CAD build for the part. Positions are in the model's coordinates, mm. Face numbers are marked on the shaded views. A direction names the side the tool comes from. Coordinates: 2 decimals unless noted, no trailing zeros. Loops run counter-clockwise (first coordinate to the right, second up) from the corner with the lowest first, then second, coordinate; pieces in that order, holes last. Notation, with made-up numbers: (24, 63.5) - (36, 63.5) arc R26 ccw to (36, 99.5) - close; hole circle Ø8 at (39.25, 65). An arc over 180 degrees is marked (long way). Put each result on its own line as item: value.
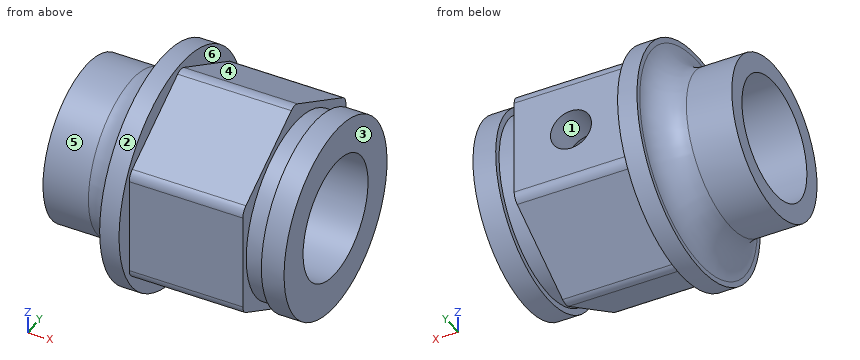
Autodesk Inventor part; units mm, degrees
ref_plane "YZ Plane" through (0, 0, 0) normal (1, 0, 0) x (0, 1, 0)
ref_plane "XZ Plane" through (0, 0, 0) normal (0, 1, 0) x (-1, 0, 0)
ref_plane "XY Plane" through (0, 0, 0) normal (0, 0, 1) x (1, 0, 0)
sketch "Sketch1" plane through (0, 0, 0) normal (1, 0, 0) x (0, 1, 0)
  circle A0 centre (0, 0) radius 7.5985
  dimension "d0" = 15.197
extrude "Extrusion1" add sketch "Sketch1" along normal blind 1.28
sketch "Sketch2" plane through (1.28, 0, 0) normal (1, 0, 0) x (0, 0, -1)
  line L0 (3.6604, 6.34) -> (7.3208, 0)
  line L1 (7.3208, 0) -> (3.6604, -6.34)
  line L2 (3.6604, -6.34) -> (-3.6604, -6.34)
  line L3 (-3.6604, -6.34) -> (-7.3208, 0)
  line L4 (-7.3208, 0) -> (-3.6604, 6.34)
  line L5 (-3.6604, 6.34) -> (3.6604, 6.34)
  point P0 (0, 0)
  point P1 (0, 6.34)
  point P2 (0, 0)
extrude "Extrusion2" add sketch "Sketch2" along normal blind 7.5
sketch "Sketch3" plane through (8.78, 0, 0) normal (1, 0, 0) x (0, 0, -1)
  circle A0 centre (0, 0) radius 5.927
  dimension "d5" = 11.854
extrude "Extrusion3" add sketch "Sketch3" along normal blind 1.22
sketch "Sketch4" plane through (10, 0, 0) normal (1, 0, 0) x (0, 0, -1)
  circle A0 centre (0, 0) radius 6.34
  line L0 (3.6604, 6.34) -> (-3.6604, 6.34)
extrude "Extrusion4" add sketch "Sketch4" along normal blind 1.5
fillet "Fillet1" radius 0.75 5 edges at (5.03, 0, -7.3208) (5.03, -6.34, -3.6604) (5.03, 0, 7.3208) (5.03, 6.34, -3.6604) (5.03, 6.34, 3.6604)
fillet "Fillet2" radius 0.75 1 edges at (5.03, -6.34, 3.6604)
sketch "Sketch5" plane through (0, 0, 0) normal (-1, 0, 0) x (0, 0, 1)
  point P0 (0, 0)
sketch "Sketch6" plane through (1.28, 6.34, 3.2274) normal (0, 1, 0) x (1, 0, 0)
  circle A0 centre (3.75, 3.2274) radius 1.3525
  point P0 (-1.28, 3.2274)
  dimension "d12" = 2.705
extrude "Extrusion5" cut sketch "Sketch6" against normal blind 6.5
sketch "Sketch7" plane through (0, 0, 0) normal (-1, 0, 0) x (0, 0, 1)
  circle A0 centre (0, 0) radius 3.2
  dimension "d15" = 6.4
sketch "Sketch8" plane through (5.03, -0.16, 0) normal (0, 1, 0) x (1, 0, 0)
  point P0 (-5.03, 0)
extrude "Extrusion6" cut sketch "Sketch7" against normal blind 11.75
sketch "Sketch9" plane through (11.5, 0, 0) normal (1, 0, 0) x (0, 0, -1)
  circle A0 centre (0, 0) radius 4
  dimension "d18" = 8
extrude "Extrusion7" cut sketch "Sketch9" against normal blind 13.75
sketch "Sketch10" plane through (0, 0, 0) normal (-1, 0, 0) x (0, 0, 1)
  circle A0 centre (0, 0) radius 4
  circle A1 centre (0, 0) radius 5.25
  dimension "d21" = 10.5
extrude "Extrusion8" add sketch "Sketch10" along normal blind 5
fillet "Fillet3" radius 2 1 edges at (0, 0, -5.25)
properties part number "_3DPrint"
Q1. Tool access for the marked faces 4, 5 and 6: list every direction of +Z, -Z, +X, -X, +Y, -Y with a clear straight run to the whole face (end or side of a thin tool).
Determined:
face 4: +Z, +X, +Y
face 5: -X
face 6: +X
Q2. Wall check: L1, parallel to Y at x = -3, z = 0; L2, parallel to Y at x = 2.5, z = 0; L3, parallel to Z at x = 6.25, y = 0. Give the ranges that are in metal, low to high. Write a range as from..to.
Determined:
L1: -5.25..-4, 4..5.25
L2: -6.34..-4, 4..6.34
L3: -7.2..-4, 4..7.2
Q3. Mould opens along Z. For the marked faces 1, 2 and 3 say: +Z half, -Z half, draft (parallel to the pull), parting line (faces both ways), or undercut.
Determined:
face 1: undercut
face 2: parting line
face 3: draft
Q4. Slice it at D-D, the plane x = 7.25. Give the cut face in (y, z) (3 decimals), then the cut area to 3 significant figures.
Determined:
outline: (-6.34, -3.227) arc R0.75 ccw to (-5.965, -3.877) - (-0.375, -7.104) arc R0.75 ccw to (0.375, -7.104) - (5.965, -3.877) arc R0.75 ccw to (6.34, -3.227) - (6.34, 3.227) arc R0.75 ccw to (5.965, 3.877) - (0.375, 7.104) arc R0.75 ccw to (-0.375, 7.104) - (-5.965, 3.877) arc R0.75 ccw to (-6.34, 3.227) - close; hole circle Ø8 at (0, 0)
area: 88.8 mm2
Q5. Pin check, flat tips, straight feed: pin 1 Ø5 at (x, z) = (9, 1) entering from +Y; pin 2 Ø1.5 at (x, y) = (-2.5, -5) entering from -Z; pin 3 Ø1.5 at (x, y) = (0, -1) entering from -Z. Stop position of each tip, or through.
Determined:
pin 1: y = 6.34
pin 2: z = -3.08
pin 3: z = -7.59
Q6. Slice it at B-B, the plane z = 0. State how many separate pieces and enclosed holes the cut face has, then the cut area to 3 significant figures.
Determined:
separate pieces: 3
enclosed holes: 0
area: 63.9 mm2
Q7. Slice it at A-A, the plane y = 0. Give the cut face in (x, z).
Determined:
outline: (-5, -5.25) - (-2, -5.25) arc R2 cw to (0, -7.25) - (0, -7.6) - (1.28, -7.6) - (1.28, -7.2) - (8.78, -7.2) - (8.78, -5.93) - (10, -5.93) - (10, -6.34) - (11.5, -6.34) - (11.5, -4) - (-5, -4) - close; (-5, 4) - (11.5, 4) - (11.5, 6.34) - (10, 6.34) - (10, 5.93) - (8.78, 5.93) - (8.78, 7.2) - (1.28, 7.2) - (1.28, 7.6) - (0, 7.6) - (0, 7.25) arc R2 cw to (-2, 5.25) - (-5, 5.25) - close
